Check sheet for the modelled part. Datum: model origin and axes. Units: mm. Give positions to 0.01 mm unless a question says otherwise; leave off trailing zeros. Order: outer loops, then holes, each group sorted by start corner. A loop starts at its lowest first (then second) coordinate and runs counter-clockwise, first axis right, second up.
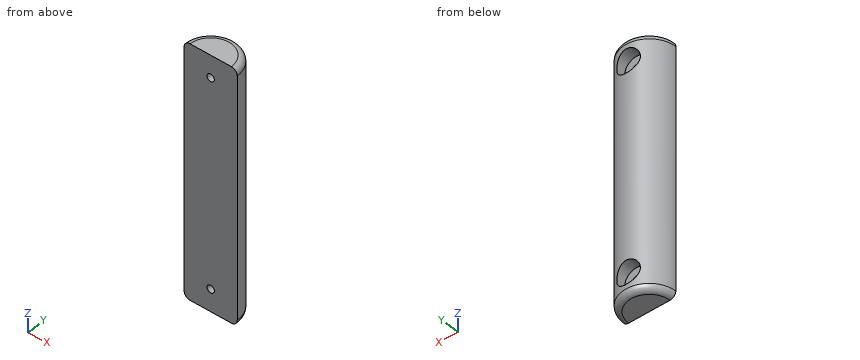
Autodesk Inventor part; units mm, degrees
ref_plane "YZ Plane" through (0, 0, 0) normal (1, 0, 0) x (0, 1, 0)
ref_plane "XZ Plane" through (0, 0, 0) normal (0, 1, 0) x (-1, 0, 0)
ref_plane "XY Plane" through (0, 0, 0) normal (0, 0, 1) x (1, 0, 0)
sketch "Sketch3" plane through (0, 0, 0) normal (0, 0, 1) x (1, 0, 0)
  line L0 (0, -1.8) -> (0, 10.8) construction
  line L1 (-12.6, 0) -> (12.6, 0) construction
  line L2 (-9, 0) -> (9, 0)
  line L3 (9, 0) -> (9, 0)
  arc A0 (9, 0) -> (-9, 0) centre (0, 0) ccw
  line L4 (-9, 0) -> (-9, 0)
  dimension "d20" = 18
  dimension "d21" = 0
extrude "Extrusion3" add sketch "Sketch3" along normal blind 85
fillet "Fillet1" radius 2 2 edges at (0, 9, 0) (0, 9, 85)
sketch "Sketch4" plane through (0, 0, 0) normal (0, 1, 0) x (-1, 0, 0)
  circle A0 centre (0, 77.5) radius 1.25
  circle A1 centre (0, 7.5) radius 1.25
  circle A2 centre (0, 7.5) radius 4
  circle A3 centre (0, 77.5) radius 4
  line L0 (9, 42.5) -> (-9, 42.5) construction
  arc A4 (-7, 85) -> (-9, 83) centre (-7, 83) ccw
  line L1 (-7, 85) -> (7, 85)
  arc A5 (9, 83) -> (7, 85) centre (7, 83) ccw
  line L2 (9, 83) -> (9, 2)
  arc A6 (7, 0) -> (9, 2) centre (7, 2) ccw
  line L3 (7, 0) -> (-7, 0)
  arc A7 (-9, 2) -> (-7, 0) centre (-7, 2) ccw
  line L4 (-9, 2) -> (-9, 83)
  point P0 (0, 0)
  dimension "d25" = 8
  dimension "d26" = 2.5
  dimension "d31" = 70
extrude "Extrusion4" cut sketch "Sketch4" along normal blind 85 contours A0 | A1 | A2 | A3
extrude "Extrusion5" add sketch "Sketch4" along normal blind 5 from surface at 0 contours A2 | A3
properties part number "BodySiliconeRubber"
Q1. Sectioned sample at A-A, the plane x = 0. Record the cut outline in (y, z).
Q2. Sectioned sample at C-C, the plane z = 38.5. Record the cut outline in (x, y), plus the area to 3 significant figures.
Q3. Material ranges on line 1 (Z direction, x = 0, y = 3.55); line 2 (Z direction, x = 0, y = 6.45); line 3 (X direction, y = 2.1, z = 77.5), recorded low to high.
Q4. Sectioned sample at D-D, the plane y = 1.25. Count the separate pieces of the cut face and the enclosed holes in it, plus the area to 3 significant figures.
Q5. Go/stop test with flat-tipped pins: P1, Ø6.5, axis at x = 1.5, z = 8.5, coming from the +Y side; P2, Ø3, axis at x = -5.5, z = 73, coming from the +Y side; P3, Ø3, axis at x = 0, z = 77.5, coming from the +Y side. Record where each tip stops, or that it passes through.
Q6. Sectioned sample at B-B, the plane z = 7.5. Record the cut outline in (x, y), plus the area to 3 significant figures.
Filled in:
1. outline: (0, 0) - (7, 0) arc R2 ccw to (9, 2) - (9, 3.5) - (5, 3.5) - (5, 6.25) - (0, 6.25) - close; (0, 8.75) - (5, 8.75) - (5, 11.5) - (9, 11.5) - (9, 73.5) - (5, 73.5) - (5, 76.25) - (0, 76.25) - close; (0, 78.75) - (5, 78.75) - (5, 81.5) - (9, 81.5) - (9, 83) arc R2 ccw to (7, 85) - (0, 85) - close
2. outline: (-9, 0) - (9, 0) arc R9 ccw to start
2. area: 127 mm2
3. line 1: z = 0 to 6.25, 8.75 to 76.25, 78.75 to 85
3. line 2: z = 0 to 3.5, 11.5 to 73.5, 81.5 to 85
3. line 3: x = -8.75 to -1.25, 1.25 to 8.75
4. separate pieces: 1
4. enclosed holes: 2
4. area: 1,500 mm2
5. P1: stops at y = 9
5. P2: stops at y = 8.06
5. P3: stops at y = 5
6. outline: (-9, 0) - (-1.25, 0) - (-1.25, 5) - (-4, 5) - (-4, 8.06) arc R9 ccw to start; (1.25, 0) - (9, 0) arc R9 ccw to (4, 8.06) - (4, 5) - (1.25, 5) - close
6. area: 85.2 mm2
